Build history of the part. All positions in model axes, mm. Face numbers are marked on the shaded views. Coordinates: 2 decimals unless noted, no trailing zeros. Write each loop counter-clockwise with the first axis right and the second up, starting at its lowest first coordinate (ties: lowest second). Pieces come first, ordered by that corner, then holes.
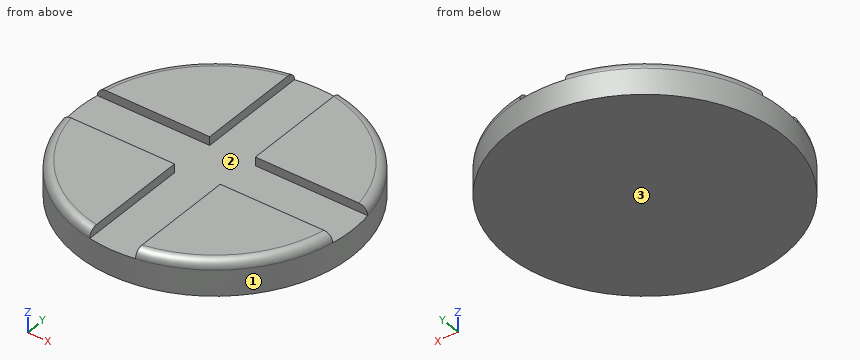
```python
from build123d import *

# Parameters (mm, degrees)
SKETCH1_R           = 4
BOSS_EXTRUDE1_DEPTH = 1
CUT_EXTRUDE1_DEPTH  = 0.25
FILLET1_R           = 0.25


with BuildPart() as part:
    # Sketch1 → Boss-Extrude1 (new body)
    with BuildSketch(Plane.XY):
        Circle(SKETCH1_R)
    extrude(amount=BOSS_EXTRUDE1_DEPTH)

    # Sketch2 → Cut-Extrude1 (cut)
    with BuildSketch(Plane.XY.offset(1)):
        Polygon((-8.106259115, 0.675521593), (-0.666748585, 0.675521593), (-0.666748585, 8.465952431), (0.666748585, 8.465952431), (0.666748585, 0.675521593), (8.106259115, 0.675521593), (8.106259115, -0.675521593), (0.666748585, -0.675521593), (0.666748585, -8.465952431), (-0.666748585, -8.465952431), (-0.666748585, -0.675521593), (-8.106259115, -0.675521593), align=None)
    extrude(amount=-CUT_EXTRUDE1_DEPTH, mode=Mode.SUBTRACT)

    # Fillet1
    fillet1_edges = [part.edges().sort_by_distance(p)[0] for p in [
        (2.825279045, 2.831571704, 1),
        (2.825279045, -2.831571704, 1),
        (-2.825279045, -2.831571704, 1),
        (-2.825279045, 2.831571704, 1),
    ]]
    fillet(fillet1_edges, radius=FILLET1_R)


solid = part.part
```
1. Saw through at B-B on y = 0. List the corners of the cut face in (x, z), plus the area to 3 significant figures.
Computed values:
outline: (-4, 0) - (4, 0) - (4, 0.75) - (-4, 0.75) - close
area: 6.00 mm2
2. Mould opens along X. For the marked faces 1, 2 and 3 say: +X half, -X half, draft (parallel to the pull), parting line (faces both ways), or undercut.
Computed values:
face 1: parting line
face 2: undercut
face 3: draft
3. Saw through at A-A on z = 0.9. List the corners of the cut face in (x, y).
Computed values:
outline: (-3.89, -0.68) arc R3.95 ccw to (-0.67, -3.89) - (-0.67, -0.68) - close; (-3.89, 0.68) - (-0.67, 0.68) - (-0.67, 3.89) arc R3.95 ccw to start; (0.67, -3.89) arc R3.95 ccw to (3.89, -0.68) - (0.67, -0.68) - close; (0.67, 0.68) - (3.89, 0.68) arc R3.95 ccw to (0.67, 3.89) - close
4. Probe line 1 along X through (y, z) = (-1, 0.8); line 2 along Z through (x, y) = (1.5, 0.5); line 3 along X through (y, z) = (-2.5, 0.85). List the from-to ranges inside material, lowest first.
Computed values:
line 1: x = -3.87 to -0.67, 0.67 to 3.87
line 2: z = 0 to 0.75
line 3: x = -3.1 to -0.67, 0.67 to 3.1
